The listing builds one solid part. Answer for the finished solid, in the listing's coordinates (mm). A direction names the side the tool comes from. Coordinates: 2 decimals unless noted, no trailing zeros. Order: outer loops, then holes, each group sorted by start corner. A loop starts at its lowest first (then second) coordinate and runs counter-clockwise, first axis right, second up. Notation, with made-up numbers: (79, 87) -> (97, 87) arc R25 cw to (97, 114) -> close; hole circle Ø7 at (42.5, 21). An arc over 180 degrees is marked (long way). Return JSON: item names as keys, results as strings.
from build123d import *

# Parameters (mm, degrees)
F0_R          = 101.6
F0_R_2        = 83.82
F1_DEPTH      = 38.1
F1_DEPTH_BACK = 38.1
F0_R_3        = 34.925
F0_R_4        = 31.115
F2_DEPTH      = 24.13
F2_DEPTH_BACK = 24.13
F3_R          = 5.08


# Not quite as in the source:
# - a length typed as a fraction of an inch, garbled in the dataset ("3 / 203.2 mm" for 3/8 in), is restored


with BuildPart() as f1:
    # F0 (on Right) → F1 (new body, two sides)
    with BuildSketch(Plane.YZ) as f1_sk:
        Circle(F0_R)
        Circle(F0_R_2, mode=Mode.SUBTRACT)
    extrude(amount=F1_DEPTH)
    extrude(f1_sk.sketch, amount=-F1_DEPTH_BACK)



with BuildPart() as f1b:
    # F0 (on Right) → F1, piece 2 (new body, two sides)
    with BuildSketch(Plane.YZ) as f1_2_sk:
        Circle(F0_R_3)
        Circle(F0_R_4, mode=Mode.SUBTRACT)
    extrude(amount=F1_DEPTH)
    extrude(f1_2_sk.sketch, amount=-F1_DEPTH_BACK)


with BuildPart() as f1_1:
    add(f1.part)

    add(f1b.part)  # F2 merges F1b
    # F0 (on Right) → F2 (join, two sides)
    with BuildSketch(Plane.YZ) as f2_sk:
        Circle(F0_R_2)
        Circle(F0_R_3, mode=Mode.SUBTRACT)
    extrude(amount=F2_DEPTH)
    extrude(f2_sk.sketch, amount=-F2_DEPTH_BACK)

    # F3
    f3_edges = [f1_1.edges().sort_by_distance(p)[0] for p in [
        (24.13, -34.925, 0),
        (24.13, -83.82, 0),
        (-24.13, -34.925, 0),
        (-24.13, -83.82, 0),
    ]]
    fillet(f3_edges, radius=F3_R)


solid = f1_1.part
1. The part is cut by section C-C on x = 14. Give the vertices of the cut face in (y, z) (3 decimals), and give its area (3 significant figures).
Answer block:
{"outline": "circle Ø203.2 at (0, 0); hole circle Ø62.23 at (0, 0)", "area": "29,400 mm2"}
2. Each of these flat-tipped pins is pushed along its axis until it touches: pin 1 Ø2 at (x, y) = (17, -11.5) entering from -Z; pin 2 Ø2 at (x, y) = (-13, -27.5) entering from +Z; pin 3 Ø6 at (x, y) = (-8.5, -49) entering from -Z. Where does it stop, or does it pass through?
Answer block:
{"pin 1": "stops at z = -101.06", "pin 2": "stops at z = 98.08", "pin 3": "stops at z = -90.59"}
3. Consider line 1 (Z direction, x = -34, y = 0) (3 decimals); line 2 (X direction, y = -72, z = 30); line 3 (Z direction, x = 21, y = 0) (3 decimals). Determine where each line is inside the solid, lowest interval first. Write a range as from..to.
Answer block:
{"line 1": "z = -101.6..-83.82, -34.925..-31.115, 31.115..34.925, 83.82..101.6", "line 2": "x = -24.13..24.13", "line 3": "z = -101.6..-31.115, 31.115..101.6"}
4. For faces 1 (the face through (33.593, -10.912, 83.107)), 2 (the face through (38.1, -31.2, -2.4)), 3 (the face through (-24.13, -36, 19)), determine the directions among +Z, -Z, +X, -X, +Y, -Y from which every point of the face is accessible in a straight line to the end or side of a thin tool.
Answer block:
{"face 1": "+X", "face 2": "+Z, -Z, +X, +Y, -Y", "face 3": "-X"}
5. Determine the mould class of faces 4 (the face through (-33.717, -10.912, 83.107)), 5 (the face through (-38.1, -31.2, -2.4)), 6 (the face through (0.533, -22.025, -99.184)) for opening direction Z: pulls with the +Z half, pulls with the -Z half, needs draft (parallel to the pull), parting line crosses it, or undercut.
Answer block:
{"face 4": "undercut", "face 5": "needs draft", "face 6": "parting line crosses it"}
6. The part is cut by section B-B on x = 33. Give the vertices of the cut face in (y, z) (3 decimals).
Answer block:
{"outline": "circle Ø203.2 at (0, 0); circle Ø69.85 at (0, 0); hole circle Ø167.64 at (0, 0); hole circle Ø62.23 at (0, 0)"}
